Geometry: final body of the model. Coordinates: model frame, mm. A direction names the side the tool comes from. Round coordinates to 2 decimals unless told otherwise and drop trailing zeros. Loops run counter-clockwise (first coordinate to the right, second up) from the corner with the lowest first, then second, coordinate; pieces in that order, holes last. Notation, with made-up numbers: M 54,-24.5 L 82,-24.5 A28 ccw 82,14.5 Z; hole C 72.25,-28.75 d5. An arc over 180 degrees is marked long. Write each question's results on one line, items separated by ' | '.
```python
from build123d import *

# Parameters (mm, degrees)
BOSS_EXTRUDE1_DEPTH = 304.8
CUT_EXTRUDE1_REACH  = 16.288


with BuildPart() as part:
    # Sketch1 → Boss-Extrude1 (new body)
    with BuildSketch(Plane(origin=(0, 0, 0), x_dir=(0, 0, -1), z_dir=(1, 0, 0))):
        with BuildLine():
            Line((-0.762, 67.29984), (12.7, 67.29984))
            Line((12.7, 67.29984), (12.7, 65.71234))
            Line((12.7, 65.71234), (0.8255, 65.71234))
            ThreePointArc((0.8255, 65.71234), (0.241783352, 65.470556648), (0, 64.88684))
            Line((0, 64.88684), (0, 0.8255))
            ThreePointArc((0, 0.8255), (0.241783352, 0.241783352), (0.8255, 0))
            Line((0.8255, 0), (12.7, 0))
            Line((12.7, 0), (12.7, -1.5875))
            Line((12.7, -1.5875), (-0.762, -1.5875))
            ThreePointArc((-0.762, -1.5875), (-1.345716648, -1.345716648), (-1.5875, -0.762))
            Line((-1.5875, -0.762), (-1.5875, 66.47434))
            ThreePointArc((-1.5875, 66.47434), (-1.345716648, 67.058056648), (-0.762, 67.29984))
        make_face()
    extrude(amount=BOSS_EXTRUDE1_DEPTH)

    # Sketch2 → Cut-Extrude1 (cut, up to next)
    with BuildSketch(Plane.XY.offset(1.5875), mode=Mode.PRIVATE) as cut_extrude1_sk1:
        with BuildLine():
            Line((32.681340962, 56.921546337), (15.411988703, 46.951081161))
            ThreePointArc((15.411988703, 46.951081161), (13.668792717, 45.207885176), (13.030738703, 42.826635176))
            Line((13.030738703, 42.826635176), (13.030738703, 22.885704824))
            ThreePointArc((13.030738703, 22.885704824), (13.668792717, 20.504454824), (15.411988703, 18.761258839))
            Line((15.411988703, 18.761258839), (32.681340962, 8.790793663))
            ThreePointArc((32.681340962, 8.790793663), (35.062590962, 8.152739649), (37.443840962, 8.790793663))
            Line((37.443840962, 8.790793663), (54.713193222, 18.761258839))
            ThreePointArc((54.713193222, 18.761258839), (56.456389207, 20.504454824), (57.094443222, 22.885704824))
            Line((57.094443222, 22.885704824), (57.094443222, 42.826635176))
            ThreePointArc((57.094443222, 42.826635176), (56.456389207, 45.207885176), (54.713193222, 46.951081161))
            Line((54.713193222, 46.951081161), (37.443840962, 56.921546337))
            ThreePointArc((37.443840962, 56.921546337), (35.062590962, 57.559600351), (32.681340962, 56.921546337))
        make_face()
    cut_extrude1_tool1 = extrude(cut_extrude1_sk1.sketch, amount=-CUT_EXTRUDE1_REACH, mode=Mode.PRIVATE) & part.part
    add(cut_extrude1_tool1.solids().sort_by_distance((35.062591, 32.85617, 1.5875))[0], mode=Mode.SUBTRACT)
    # Sketch2 → Cut-Extrude1 (cut, up to next)
    with BuildSketch(Plane.XY.offset(1.5875), mode=Mode.PRIVATE) as cut_extrude1_sk2:
        with BuildLine():
            Line((91.350045481, 56.921546337), (74.080693222, 46.951081161))
            ThreePointArc((74.080693222, 46.951081161), (72.337497236, 45.207885176), (71.699443222, 42.826635176))
            Line((71.699443222, 42.826635176), (71.699443222, 22.885704824))
            ThreePointArc((71.699443222, 22.885704824), (72.337497236, 20.504454824), (74.080693222, 18.761258839))
            Line((74.080693222, 18.761258839), (91.350045481, 8.790793663))
            ThreePointArc((91.350045481, 8.790793663), (93.731295481, 8.152739649), (96.112545481, 8.790793663))
            Line((96.112545481, 8.790793663), (113.381897741, 18.761258839))
            ThreePointArc((113.381897741, 18.761258839), (115.125093726, 20.504454824), (115.763147741, 22.885704824))
            Line((115.763147741, 22.885704824), (115.763147741, 42.826635176))
            ThreePointArc((115.763147741, 42.826635176), (115.125093726, 45.207885176), (113.381897741, 46.951081161))
            Line((113.381897741, 46.951081161), (96.112545481, 56.921546337))
            ThreePointArc((96.112545481, 56.921546337), (93.731295481, 57.559600351), (91.350045481, 56.921546337))
        make_face()
    cut_extrude1_tool2 = extrude(cut_extrude1_sk2.sketch, amount=-CUT_EXTRUDE1_REACH, mode=Mode.PRIVATE) & part.part
    add(cut_extrude1_tool2.solids().sort_by_distance((93.731295, 32.85617, 1.5875))[0], mode=Mode.SUBTRACT)
    # Sketch2 → Cut-Extrude1 (cut, up to next)
    with BuildSketch(Plane.XY.offset(1.5875), mode=Mode.PRIVATE) as cut_extrude1_sk3:
        with BuildLine():
            Line((150.01875, 56.921546337), (132.749397741, 46.951081161))
            ThreePointArc((132.749397741, 46.951081161), (131.006201755, 45.207885176), (130.368147741, 42.826635176))
            Line((130.368147741, 42.826635176), (130.368147741, 22.885704824))
            ThreePointArc((130.368147741, 22.885704824), (131.006201755, 20.504454824), (132.749397741, 18.761258839))
            Line((132.749397741, 18.761258839), (150.01875, 8.790793663))
            ThreePointArc((150.01875, 8.790793663), (152.4, 8.152739649), (154.78125, 8.790793663))
            Line((154.78125, 8.790793663), (172.050602259, 18.761258839))
            ThreePointArc((172.050602259, 18.761258839), (173.793798245, 20.504454824), (174.431852259, 22.885704824))
            Line((174.431852259, 22.885704824), (174.431852259, 42.826635176))
            ThreePointArc((174.431852259, 42.826635176), (173.793798245, 45.207885176), (172.050602259, 46.951081161))
            Line((172.050602259, 46.951081161), (154.78125, 56.921546337))
            ThreePointArc((154.78125, 56.921546337), (152.4, 57.559600351), (150.01875, 56.921546337))
        make_face()
    cut_extrude1_tool3 = extrude(cut_extrude1_sk3.sketch, amount=-CUT_EXTRUDE1_REACH, mode=Mode.PRIVATE) & part.part
    add(cut_extrude1_tool3.solids().sort_by_distance((152.4, 32.85617, 1.5875))[0], mode=Mode.SUBTRACT)
    # Sketch2 → Cut-Extrude1 (cut, up to next)
    with BuildSketch(Plane.XY.offset(1.5875), mode=Mode.PRIVATE) as cut_extrude1_sk4:
        with BuildLine():
            Line((208.687454519, 56.921546337), (191.418102259, 46.951081161))
            ThreePointArc((191.418102259, 46.951081161), (189.674906274, 45.207885176), (189.036852259, 42.826635176))
            Line((189.036852259, 42.826635176), (189.036852259, 22.885704824))
            ThreePointArc((189.036852259, 22.885704824), (189.674906274, 20.504454824), (191.418102259, 18.761258839))
            Line((191.418102259, 18.761258839), (208.687454519, 8.790793663))
            ThreePointArc((208.687454519, 8.790793663), (211.068704519, 8.152739649), (213.449954519, 8.790793663))
            Line((213.449954519, 8.790793663), (230.719306778, 18.761258839))
            ThreePointArc((230.719306778, 18.761258839), (232.462502764, 20.504454824), (233.100556778, 22.885704824))
            Line((233.100556778, 22.885704824), (233.100556778, 42.826635176))
            ThreePointArc((233.100556778, 42.826635176), (232.462502764, 45.207885176), (230.719306778, 46.951081161))
            Line((230.719306778, 46.951081161), (213.449954519, 56.921546337))
            ThreePointArc((213.449954519, 56.921546337), (211.068704519, 57.559600351), (208.687454519, 56.921546337))
        make_face()
    cut_extrude1_tool4 = extrude(cut_extrude1_sk4.sketch, amount=-CUT_EXTRUDE1_REACH, mode=Mode.PRIVATE) & part.part
    add(cut_extrude1_tool4.solids().sort_by_distance((211.068705, 32.85617, 1.5875))[0], mode=Mode.SUBTRACT)
    # Sketch2 → Cut-Extrude1 (cut, up to next)
    with BuildSketch(Plane.XY.offset(1.5875), mode=Mode.PRIVATE) as cut_extrude1_sk5:
        with BuildLine():
            Line((267.356159038, 56.921546337), (250.086806778, 46.951081161))
            ThreePointArc((250.086806778, 46.951081161), (248.343610793, 45.207885176), (247.705556778, 42.826635176))
            Line((247.705556778, 42.826635176), (247.705556778, 22.885704824))
            ThreePointArc((247.705556778, 22.885704824), (248.343610793, 20.504454824), (250.086806778, 18.761258839))
            Line((250.086806778, 18.761258839), (267.356159038, 8.790793663))
            ThreePointArc((267.356159038, 8.790793663), (269.737409038, 8.152739649), (272.118659038, 8.790793663))
            Line((272.118659038, 8.790793663), (289.388011297, 18.761258839))
            ThreePointArc((289.388011297, 18.761258839), (291.131207283, 20.504454824), (291.769261297, 22.885704824))
            Line((291.769261297, 22.885704824), (291.769261297, 42.826635176))
            ThreePointArc((291.769261297, 42.826635176), (291.131207283, 45.207885176), (289.388011297, 46.951081161))
            Line((289.388011297, 46.951081161), (272.118659038, 56.921546337))
            ThreePointArc((272.118659038, 56.921546337), (269.737409038, 57.559600351), (267.356159038, 56.921546337))
        make_face()
    cut_extrude1_tool5 = extrude(cut_extrude1_sk5.sketch, amount=-CUT_EXTRUDE1_REACH, mode=Mode.PRIVATE) & part.part
    add(cut_extrude1_tool5.solids().sort_by_distance((269.737409, 32.85617, 1.5875))[0], mode=Mode.SUBTRACT)


solid = part.part
```
1. Section A-A (y = 35.5). Output: boundary loops of the cut face in (x, z), then the cut area to 3 significant figures.
Answer key:
outline: M 0,0 L 13.03,0 L 13.03,1.59 L 0,1.59 Z; M 57.09,0 L 71.7,0 L 71.7,1.59 L 57.09,1.59 Z; M 115.76,0 L 130.37,0 L 130.37,1.59 L 115.76,1.59 Z; M 174.43,0 L 189.04,0 L 189.04,1.59 L 174.43,1.59 Z; M 233.1,0 L 247.71,0 L 247.71,1.59 L 233.1,1.59 Z; M 291.77,0 L 304.8,0 L 304.8,1.59 L 291.77,1.59 Z | area: 134 mm²
2. Section D-D (y = 12.5). Output: boundary loops of the cut face in (x, z).
Answer key:
outline: M 0,0 L 26.26,0 L 26.26,1.59 L 0,1.59 Z; M 43.87,0 L 84.93,0 L 84.93,1.59 L 43.87,1.59 Z; M 102.54,0 L 143.59,0 L 143.59,1.59 L 102.54,1.59 Z; M 161.21,0 L 202.26,0 L 202.26,1.59 L 161.21,1.59 Z; M 219.87,0 L 260.93,0 L 260.93,1.59 L 219.87,1.59 Z; M 278.54,0 L 304.8,0 L 304.8,1.59 L 278.54,1.59 Z
3. Access query for faces 5 (the face through (104.63, 13.71, 0.8)), 6 (the face through (116, 33, 0)), 7 (the face through (150, 67.3, -6)). Directions: +Z, -Z, +X, -X, +Y, -Y. A direction counts if a zero-diameter tool reaches every point of the face in a straight line with its end or side. Return the directions, or none.
Answer key:
face 5: +Z, -Z | face 6: -Z, +X, -X | face 7: +Z, -Z, +X, -X, +Y
4. Ray query, probe 1 along Y at (x, z) = (28.5, -2.5); probe 2 along X at (y, z) = (14, 0.25); probe 3 along Z at (x, y) = (226, 3). Return the intervals inside material, ascending.
Answer key:
probe 1: y = -1.59 to 0, 65.71 to 67.3 | probe 2: x = 0 to 23.66, 46.47 to 82.33, 105.14 to 141, 163.8 to 199.66, 222.47 to 258.33, 281.14 to 304.8 | probe 3: z = 0 to 1.59
5. Draft query along Y for faces 1 (the face through (0, 33, 0.2)), 2 (the face through (150, -1.588, -6)), 3 (the face through (258.601, 13.846, 0.805)), 4 (the face through (46.199, 51.867, 0.805)). Return one class per face: pulls with the +Y half, pulls with the -Y half, needs draft (parallel to the pull), parting line crosses it, or undercut.
Answer key:
face 1: needs draft | face 2: pulls with the -Y half | face 3: undercut | face 4: undercut
6. Section B-B (z = -5). Output: boundary loops of the cut face in (x, y).
Answer key:
outline: M 0,-1.59 L 304.8,-1.59 L 304.8,0 L 0,0 Z; M 0,65.71 L 304.8,65.71 L 304.8,67.3 L 0,67.3 Z
7. Section C-C (x = 99). Output: boundary loops of the cut face in (y, z).
Answer key:
outline: M -1.59,-12.7 L 0,-12.7 L 0,-0.83 A0.83 cw 0.83,0 L 10.46,0 L 10.46,1.59 L -0.76,1.59 A0.83 ccw -1.59,0.76 Z; M 55.25,0 L 64.89,0 A0.83 cw 65.71,-0.83 L 65.71,-12.7 L 67.3,-12.7 L 67.3,0.76 A0.83 ccw 66.47,1.59 L 55.25,1.59 Z
8. Pin query (flat end, axial travel): P1, Ø6, axis at x = 230.5, y = 41.5, coming from the -Z side. Return the tip coordinate at first contact, or that it passes through.
Answer key:
P1: stops at z = 0
